Here's how the part is built. I have some questions about the finished solid (model axes, mm). Face numbers are marked on the shaded views. A direction names the side the tool comes from. Coordinates: 2 decimals unless noted, no trailing zeros. Loops run counter-clockwise (first coordinate to the right, second up) from the corner with the lowest first, then second, coordinate; pieces in that order, holes last. Notation, with made-up numbers: M 77,-4.75 L 96,-4.75 A16 cw 96,15.25 Z; hole C 59.25,12.5 d4. An arc over 180 degrees is marked long. Use CSV: the item, a comma, the result in double quotes. Start each with the question number.
Q1. Which directions (+Z, -Z, +X, -X, +Y, -Y) give clear straight access to the entire face, cutting with the end or side of a thin tool? Please do the marked faces 1 and 2.
Q2. If we section it at D-D (z = 3): Please give me the cut outline in (x, y), and give its area (3 significant figures).
Q3. For pin 1 Ø5 at (x, y) = (-27.5, -7) entering from +Z; pin 2 Ø6 at (y, z) = (-10, 6.5) entering from +X; pin 3 Ø4 at (y, z) = (-10, 14.5) entering from +X; pin 4 Ø10 at (y, z) = (-0.5, 5.5) entering from +X, each with a flat end and sliding along its axis, tell me the tip position at first contact or that it passes through.
Q4. If we section it at A-A (z = 16.5): Please give me the cut outline in (x, y), and give its area (3 significant figures).
Q5. If we section it at B-B (x = -24): Please give me the cut outline in (y, z).
Q6. If we mould it in two halves opening along X, with no side actions, what happens to the marked faces 3, 4 and 5? For each: +X half, -X half, draft (parallel to the pull), parting line (faces both ways), or undercut.
Q7. If we section it at C-C (y = -1): Please give me the cut outline in (x, z).
Q8. Please list where these lines run through material, in increasing order: probe 1 along X at (y, z) = (-15, 10.75); probe 2 along Y at (x, z) = (-35, 9.75); probe 3 along X at (y, z) = (6, 2.5). Write a range as [from, to].
from build123d import *

# Parameters (mm, degrees)
SKETCH_1_W          = 86
SKETCH_1_H          = 44.4
EXTRUDE_1_DEPTH     = 19.6
EXTRUDE_2_DEPTH     = 5
SKETCH_3_W          = 26.733333333
SKETCH_3_H          = 42
SKETCH_3_W_2        = 27.333333334
CUT_EXTRUDE_1_DEPTH = 18.4
FILLET_1_R          = 3


with BuildPart() as part:
    # Эскиз1 → Бобышка-Вытянуть1 (new body)
    with BuildSketch(Plane.XY):
        Rectangle(SKETCH_1_W, SKETCH_1_H)
    extrude(amount=EXTRUDE_1_DEPTH)

    # Эскиз2 → Бобышка-Вытянуть2 (add)
    with BuildSketch(Plane.XY):
        with BuildLine():
            Line((43, 17.2), (43, 13.108775687))
            ThreePointArc((43, 13.108775687), (53.273546839, 0), (43, -13.108775687))
            Line((43, -13.108775687), (43, -17.2))
            ThreePointArc((43, -17.2), (57.273546839, 0), (43, 17.2))
        make_face()
    extrude(amount=EXTRUDE_2_DEPTH)

    # Эскиз3 → Вырез-Вытянуть1 (cut)
    with BuildSketch(Plane.XY.offset(19.6)):
        with Locations((-28.033333334, 0)):
            Rectangle(SKETCH_3_W, SKETCH_3_H)
        with Locations((0.2, 0)):
            Rectangle(SKETCH_3_W_2, SKETCH_3_H)
        with Locations((28.433333334, 0)):
            Rectangle(SKETCH_3_W, SKETCH_3_H)
    extrude(amount=-CUT_EXTRUDE_1_DEPTH, mode=Mode.SUBTRACT)

    # Скругление1
    fillet_1_edges = [part.edges().sort_by_distance(p)[0] for p in [
        (-41.4, 21, 10.4),
        (-41.4, -21, 10.4),
        (-43, -22.2, 9.8),
        (-43, 22.2, 9.8),
    ]]
    fillet(fillet_1_edges, radius=FILLET_1_R)


solid = part.part
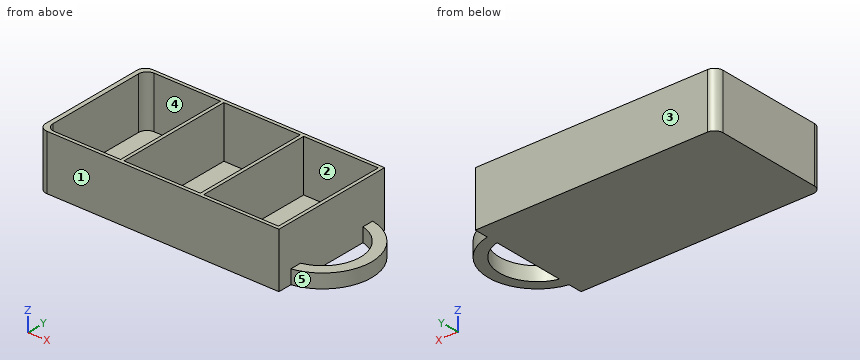
Results below:
1,face 1,"+Z, -Z, +X, -X, -Y"
1,face 2,"+Z"
2,outline,"M -43,-19.2 A3 ccw -40,-22.2 L 43,-22.2 L 43,-17.2 A17.5 ccw 43,17.2 L 43,22.2 L -40,22.2 A3 ccw -43,19.2 Z; hole M -41.4,-18 A3 ccw -38.4,-21 L -14.67,-21 L -14.67,21 L -38.4,21 A3 ccw -41.4,18 Z; hole M -13.47,-21 L 13.87,-21 L 13.87,21 L -13.47,21 Z; hole M 15.07,-21 L 41.8,-21 L 41.8,21 L 15.07,21 Z; hole M 43,-13.11 A13.5 ccw 43,13.11 Z"
2,area,"594 mm^2"
3,pin 1,"z = 1.2"
3,pin 2,"x = 55.63"
3,pin 3,"x = 43"
3,pin 4,"x = 57.27"
4,outline,"M -43,-19.2 A3 ccw -40,-22.2 L 43,-22.2 L 43,22.2 L -40,22.2 A3 ccw -43,19.2 Z; hole M -41.4,-18 A3 ccw -38.4,-21 L -14.67,-21 L -14.67,21 L -38.4,21 A3 ccw -41.4,18 Z; hole M -13.47,-21 L 13.87,-21 L 13.87,21 L -13.47,21 Z; hole M 15.07,-21 L 41.8,-21 L 41.8,21 L 15.07,21 Z"
4,area,"425 mm^2"
5,outline,"M -22.2,0 L 22.2,0 L 22.2,19.6 L 21,19.6 L 21,1.2 L -21,1.2 L -21,19.6 L -22.2,19.6 Z"
6,face 3,"draft"
6,face 4,"undercut"
6,face 5,"+X half"
7,outline,"M -43,0 L 43,0 L 43,19.6 L 41.8,19.6 L 41.8,1.2 L 15.07,1.2 L 15.07,19.6 L 13.87,19.6 L 13.87,1.2 L -13.47,1.2 L -13.47,19.6 L -14.67,19.6 L -14.67,1.2 L -41.4,1.2 L -41.4,19.6 L -43,19.6 Z; M 53.24,0 L 57.24,0 L 57.24,5 L 53.24,5 Z"
8,probe 1,"[-43, -41.4], [-14.67, -13.47], [13.87, 15.07], [41.8, 43]"
8,probe 2,"[-22.2, -21], [21, 22.2]"
8,probe 3,"[-43, -41.4], [-14.67, -13.47], [13.87, 15.07], [41.8, 43], [51.87, 56.21]"
